Part model, mm, in its own coordinate system. Face numbers are marked on the shaded views. A direction names the side the tool comes from. Coordinates: 2 decimals unless noted, no trailing zeros. Order: outer loops, then holes, each group sorted by start corner. A loop starts at its lowest first (then second) coordinate and runs counter-clockwise, first axis right, second up. Notation, with made-up numbers: (-31.5, 65) - (-12.5, 65) arc R30 ccw to (-12.5, 99) - close; hole circle Ø10 at (38, 47). An arc over 180 degrees is marked (long way). Use a Markdown table: item, result. Add a question column.
1) Two-plate mould, pull along X, no slides. Class the marked faces 4, 5 and 6: +X half, -X half, draft (parallel to the pull), parting line (faces both ways), or undercut.
2) Drop flat-ended pins along their axis: P1, Ø5, axis at x = 50.5, z = 2, coming from the +Y side; P2, Ø21, axis at y = 45.5, z = -12.5, coming from the -X side; P3, Ø9, axis at y = 44.76, z = 0, coming from the +X side. Give the stop position or say it passes through.
3) Saw through at A-A on y = 24. List the corners of the cut face in (x, z), then the cut area to 3 significant figures.
4) Saw through at C-C on x = -18.5. List the corners of the cut face in (y, z), then the cut area to 3 significant figures.
5) Wall check: L1, parallel to Y at x = -10, z = 0; L2, parallel to X at y = 33, z = 12; L3, parallel to Y at x = 25, z = -21. Give the ranges that are in metal, low to high. Write a range as [from, to].
6) Tool access for the marked faces 1, 2 and 3: list every direction of +Z, -Z, +X, -X, +Y, -Y with a clear straight run to the whole face (end or side of a thin tool).
7) Saw through at B-B on x = 25. List the corners of the cut face in (y, z).
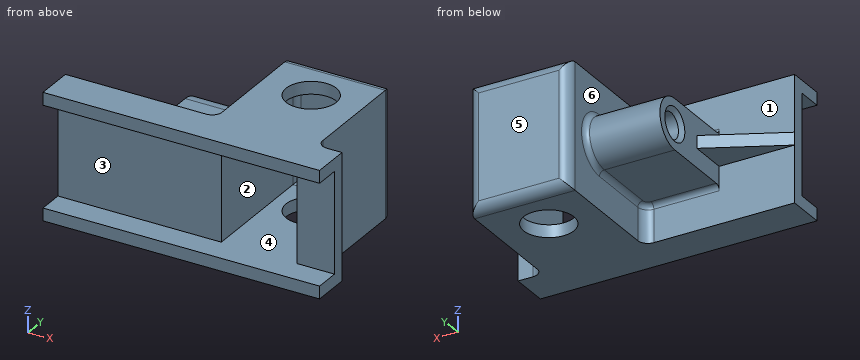
```python
from build123d import *

# Parameters (mm, degrees)
SKETCH1_W                         = 110
SKETCH1_H                         = 15
BOSS_EXTRUDE1_DEPTH               = 25
SKETCH2_W                         = 40
SKETCH2_H                         = 10
CUT_EXTRUDE1_DEPTH                = 114.798066767
SKETCH3_W                         = 40
SKETCH3_H                         = 50
SKETCH3_R                         = 10
BOSS_EXTRUDE2_DEPTH               = 50
FILLET1_R                         = 4
CUT_EXTRUDE2_DEPTH                = 20
FILLET2_R                         = 2
BOSS_EXTRUDE3_DEPTH               = 30
RIB2_REACH                        = 90.741
SKETCH7_WALL_W                    = 213.023413156
SKETCH7_WALL_H                    = 5
FILLET3_R                         = 2
FILLET4_R                         = 4
TAP_DRILL_FOR_M12X1_75_TAP1_D     = 10.2
TAP_DRILL_FOR_M12X1_75_TAP1_DEPTH = 22
TAP_DRILL_FOR_M12X1_75_TAP1_TIP   = 3.064389157


with BuildPart() as part:
    # Sketch1 → Boss-Extrude1 (new, symmetric)
    with BuildSketch(Plane.XY):
        with Locations((0, 7.5)):
            Rectangle(SKETCH1_W, SKETCH1_H)
    extrude(amount=BOSS_EXTRUDE1_DEPTH, both=True)

    # Sketch2 → Cut-Extrude1 (cut, through all)
    with BuildSketch(Plane(origin=(55, 0, 0), x_dir=(0, 0, -1), z_dir=(1, 0, 0))):
        with Locations((0, 5)):
            Rectangle(SKETCH2_W, SKETCH2_H)
    extrude(amount=-CUT_EXTRUDE1_DEPTH, mode=Mode.SUBTRACT)

    # Sketch3 → Boss-Extrude2 (add)
    with BuildSketch(Plane.XY.offset(25)):
        with Locations((25, 40)):
            Rectangle(SKETCH3_W, SKETCH3_H)
        with Locations((25, 45)):
            Circle(SKETCH3_R, mode=Mode.SUBTRACT)
    extrude(amount=-BOSS_EXTRUDE2_DEPTH)

    # Fillet1
    fillet1_edges = [part.edges().sort_by_distance(p)[0] for p in [
        (25, 65, -25),
        (5, 65, 0),
        (45, 65, 0),
        (45, 15, 0),
        (25, 65, 25),
    ]]
    fillet(fillet1_edges, radius=FILLET1_R)

    # Sketch5 → Cut-Extrude2 (cut, symmetric)
    with BuildSketch(Plane.XY):
        with BuildLine():
            Line((10, 10), (40, 10))
            Line((40, 10), (40, 58))
            ThreePointArc((40, 58), (39.414213562, 59.414213562), (38, 60))
            Line((38, 60), (12, 60))
            ThreePointArc((12, 60), (10.585786438, 59.414213562), (10, 58))
            Line((10, 58), (10, 10))
        make_face()
    extrude(amount=CUT_EXTRUDE2_DEPTH, both=True, mode=Mode.SUBTRACT)

    # Fillet2
    # the kernel refuses this fillet: 2 mm, written as the material it adds along each edge
    with BuildSketch(Plane(origin=(43, 60, 20), x_dir=(0, -1, 0), z_dir=(-1, 0, 0))) as fillet2_piece_1:
        with BuildLine():
            CenterArc((FILLET2_R, -FILLET2_R), FILLET2_R, 90, 90)
            Line((0, -FILLET2_R), (0, 0))
            Line((0, 0), (FILLET2_R, 0))
        make_face()
    extrude(amount=36)
    with BuildSketch(Plane(origin=(43, 60, -20), x_dir=(0, -1, 0), z_dir=(-1, 0, 0))) as fillet2_piece_2:
        with BuildLine():
            CenterArc((FILLET2_R, FILLET2_R), FILLET2_R, 180, 90)
            Line((0, FILLET2_R), (0, 0))
            Line((0, 0), (FILLET2_R, 0))
        make_face()
    extrude(amount=36)

    # Sketch6 → Boss-Extrude3 (add)
    with BuildSketch(Plane.ZY.offset(-5)):
        with BuildLine():
            Line((-10, 15), (10, 15))
            Line((10, 15), (10, 44.76267782))
            ThreePointArc((10, 44.76267782), (0, 54.76267782), (-10, 44.76267782))
            Line((-10, 44.76267782), (-10, 15))
        make_face()
    extrude(amount=BOSS_EXTRUDE3_DEPTH)

    # Sketch7 wall → Rib2 (add, up to next)
    with BuildSketch(Plane(origin=(-40, 22.5, 0), x_dir=(-0.894427191, -0.4472135955, 0), z_dir=(0.4472135955, -0.894427191, 0)), mode=Mode.PRIVATE) as rib2_sk1:
        Rectangle(SKETCH7_WALL_W, SKETCH7_WALL_H)
    rib2_tool1 = extrude(rib2_sk1.sketch, amount=RIB2_REACH, mode=Mode.PRIVATE) - part.part
    add(rib2_tool1.solids().sort_by_distance((-40, 22.5, 0))[0])

    # Fillet3
    fillet3_edges = [part.edges().sort_by_distance(p)[0] for p in [
        (5, 29.88133891, -10),
        (-10, 15, -10),
        (5, 29.88133891, 10),
        (-10, 15, 10),
        (5, 54.76267782, 0),
    ]]
    fillet(fillet3_edges, radius=FILLET3_R)

    # Fillet4
    # the kernel refuses this fillet: 4 mm, written as the material it adds along each edge
    with BuildSketch(Plane(origin=(1, 19, -10), x_dir=(0, -1, 0), z_dir=(-1, 0, 0))) as fillet4_piece_1:
        with BuildLine():
            CenterArc((2, -2), 2, 0, 90)
            Line((4, -2), (4, 0))
            Line((4, 0), (2, 0))
        make_face()
    revolve(axis=Axis((1, 19, -10), (0, 0, 1)), revolution_arc=90)
    with BuildSketch(Plane(origin=(1, 19, 10), x_dir=(1, 0, 0), z_dir=(0, 1, 0))) as fillet4_piece_2:
        with BuildLine():
            CenterArc((2, -2), 2, 0, 90)
            Line((4, -2), (4, 0))
            Line((4, 0), (2, 0))
        make_face()
    revolve(axis=Axis((1, 19, 10), (0, 0, -1)), revolution_arc=90)
    with BuildSketch(Plane(origin=(5, 15, 25), x_dir=(-1, 0, 0), z_dir=(0, 0, -1)), Plane(origin=(5, 15, -10), x_dir=(-1, 0, 0), z_dir=(0, 0, -1))) as fillet4_piece_3:
        with BuildLine():
            CenterArc((FILLET4_R, FILLET4_R), FILLET4_R, 180, 90)
            Line((0, FILLET4_R), (0, 0))
            Line((0, 0), (FILLET4_R, 0))
        make_face()
    extrude(amount=15)

    # Tap Drill for M12x1.75 Tap1
    with Locations(Plane(origin=(-25, 44.76267782, 0), x_dir=(0, -1, 0), z_dir=(-1, 0, 0))):
        with Locations((0, 0)):
            Hole(TAP_DRILL_FOR_M12X1_75_TAP1_D / 2, depth=TAP_DRILL_FOR_M12X1_75_TAP1_DEPTH)
            with Locations((0, 0, -(TAP_DRILL_FOR_M12X1_75_TAP1_DEPTH + TAP_DRILL_FOR_M12X1_75_TAP1_TIP / 2))):  # 118° drill point
                Cone(0, TAP_DRILL_FOR_M12X1_75_TAP1_D / 2, TAP_DRILL_FOR_M12X1_75_TAP1_TIP, mode=Mode.SUBTRACT)

    # Chamfer3: read off the stored shape, not the designer's step
    # Chamfer3 outline → Chamfer3 (revolve, cut)
    with BuildSketch(Plane(origin=(0, 44.76267782, 0), x_dir=(0, 1, 0), z_dir=(0, 0, -1))):
        Polygon((6.7, -25), (5.1, -23.4), (5.1, -25), align=None)
    revolve(axis=Axis((0, 44.76267782, 0), (1, 0, 0)), mode=Mode.SUBTRACT)


solid = part.part
```
Results are:
| question | item | result |
|---|---|---|
| 1 | face 4 | undercut |
| 1 | face 5 | draft |
| 1 | face 6 | -X half |
| 2 | P1 | y = 15.13 |
| 2 | P2 | x = -25 |
| 2 | P3 | x = 45 |
| 3 | outline | (-37, -2.5) - (-25, -2.5) - (-25, -10) - (3, -10) arc R2 cw to (5, -12) - (5, -25) - (45, -25) - (45, 25) - (5, 25) - (5, 12) arc R2 cw to (3, 10) - (-25, 10) - (-25, 2.5) - (-37, 2.5) - close; hole (10, -20) - (40, -20) - (40, 20) - (10, 20) - close |
| 3 | area | 1,460 mm2 |
| 4 | outline | (0, -25) - (15, -25) - (15, -12) arc R2 cw to (17, -10) - (44.76, -10) arc R10 ccw to (44.76, 10) - (17, 10) arc R2 cw to (15, 12) - (15, 25) - (0, 25) - (0, 20) - (10, 20) - (10, -20) - (0, -20) - close; hole circle Ø10.2 at (44.76, 0) |
| 4 | area | 1,020 mm2 |
| 5 | L1 | [10, 39.66], [49.86, 54.76] |
| 5 | L2 | [5, 10], [40, 45] |
| 5 | L3 | [0, 35], [55, 65] |
| 6 | face 1 | +Z, -X, +Y |
| 6 | face 2 | -Y |
| 6 | face 3 | +X, -X, -Y |
| 7 | outline | (0, -25) - (35, -25) - (35, -20) - (0, -20) - close; (0, 20) - (35, 20) - (35, 25) - (0, 25) - close; (55, -25) - (61, -25) arc R4 ccw to (65, -21) - (65, 21) arc R4 ccw to (61, 25) - (55, 25) - (55, 20) - (58, 20) arc R2 cw to (60, 18) - (60, -18) arc R2 cw to (58, -20) - (55, -20) - close |
